For this review, take the finished solid that the model builds, in its own axes (mm). A direction names the side the tool comes from. Round coordinates to 2 decimals unless told otherwise and drop trailing zeros. Order: outer loops, then holes, each group sorted by start corner. A loop starts at its lowest first (then second) coordinate and runs counter-clockwise, first axis right, second up. Notation, with made-up numbers: M -1,8.25 L 38,8.25 A32 ccw 38,38.25 Z; hole C -3.75,-5 d3. An arc over 180 degrees is marked long. Answer in a Markdown table with one row per item. Add a question column.
```python
from build123d import *

# Parameters (mm, degrees)
SKETCH1_W           = 260.35
SKETCH1_H           = 260.35
SKETCH1_W_2         = 254
SKETCH1_H_2         = 254
BOSS_EXTRUDE1_DEPTH = 330.2
SKETCH1_2_W         = 260.35
SKETCH1_2_H         = 260.35
BOSS_EXTRUDE2_DEPTH = 3.175


with BuildPart() as part:
    # Sketch1 → Boss-Extrude1 (new body)
    with BuildSketch(Plane.XY):
        with Locations((127, 127)):
            Rectangle(SKETCH1_W, SKETCH1_H)
        with Locations((127, 127)):
            Rectangle(SKETCH1_W_2, SKETCH1_H_2, mode=Mode.SUBTRACT)
    extrude(amount=BOSS_EXTRUDE1_DEPTH)

    # Sketch1<2> → Boss-Extrude2 (add)
    with BuildSketch(Plane.XY):
        with Locations((127, 127)):
            Rectangle(SKETCH1_2_W, SKETCH1_2_H)
    extrude(amount=-BOSS_EXTRUDE2_DEPTH)


solid = part.part
```
1. Clearance check with a flat-ended pin moving along its axis: pin 1 Ø5 at (x, y) = (185, 87) entering from +Z. State where the tip first meets the part, or that it passes through.
2. To check wall thickness, follow probe 1 along Y at (x, z) = (144, 87) (3 decimals); probe 2 along Z at (x, y) = (29.5, 174.5) (3 decimals). State the ranges of each line that lie inside material, in increasing order. Write a range as [from, to].
3. Consider section B-B on y = 187. Write out the cut boundary in (x, z) (3 decimals), plus the area to 3 significant figures.
4. Consider section A-A on z = 273. Write out the cut boundary in (x, y) (3 decimals).
5. The part is to be moulded in two halves that separate along X. For faces 1 (the flat face through (125, 254, 163)), 2 (the flat face through (257.175, 125, 166)), 3 (the flat face through (-3.175, 125, 166)), say which applies: pulls with the +X half, pulls with the -X half, needs draft (parallel to the pull), parting line crosses it, or undercut.
6. For faces 4 (the flat face through (125, 129, 0)), 5 (the flat face through (125, -3.175, 166)), list the 3-axis set-ups (+Z, -Z, +X, -X, +Y, -Y) from which the entire face can be reached by the end or side of a thin tool; tool diameter is ignored.
Solved:
| question | item | result |
|---|---|---|
| 1 | pin 1 | stops at z = 0 |
| 2 | probe 1 | y = [-3.175, 0], [254, 257.175] |
| 2 | probe 2 | z = [-3.175, 0] |
| 3 | outline | M -3.175,-3.175 L 257.175,-3.175 L 257.175,330.2 L 254,330.2 L 254,0 L 0,0 L 0,330.2 L -3.175,330.2 Z |
| 3 | area | 2,920 mm^2 |
| 4 | outline | M -3.175,-3.175 L 257.175,-3.175 L 257.175,257.175 L -3.175,257.175 Z; hole M 0,0 L 254,0 L 254,254 L 0,254 Z |
| 5 | face 1 | undercut |
| 5 | face 2 | pulls with the +X half |
| 5 | face 3 | pulls with the -X half |
| 6 | face 4 | +Z |
| 6 | face 5 | +Z, -Z, +X, -X, -Y |
